The model under review builds one solid part; all positions refer to its coordinate system, in mm. Face numbers are marked on the shaded views. Round coordinates to 2 decimals unless told otherwise and drop trailing zeros. Order: outer loops, then holes, each group sorted by start corner. A loop starts at its lowest first (then second) coordinate and runs counter-clockwise, first axis right, second up. Notation, with made-up numbers: M 18.5,-18.5 L 76.5,-18.5 A31 ccw 76.5,9.5 Z; hole C -31,63.5 d1. An arc over 180 degrees is marked long. Use a Markdown table: item, result. Add a question column.
1. The part is to be moulded in two halves that separate along Y. For the marked faces 1 and 2, say which applies: +Y half, -Y half, draft (parallel to the pull), parting line (faces both ways), or undercut.
2. Consider section A-A on z = 0. State the section outline as (x, y) points.
3. Consider section C-C on y = 12. State the section outline as (x, z) points.
4. Consider section B-B on x = -6. State the section outline as (y, z) points.
5. Insertion check: P1, Ø4, axis at x = 44.5, y = 20, coming from the -Z side; P2, Ø1.2, axis at x = -65.5, y = 2.5, coming from the +Z side; P3, Ø10, axis at x = 21.5, z = 1, coming from the +Y side; P4, Ø10, axis at y = 20, z = 1.5, coming from the -X side. Each pin has a flat end and moves straight along its axis. Give the tip position at first contact, or say it passes through.
6. To check wall thickness, follow probe 1 along X at (y, z) = (3, 0); probe 2 along Y at (x, z) = (41.5, -8.5); probe 3 along Z at (x, y) = (-49, 18). State the ranges of each line that lie inside material, in increasing order.
from build123d import *

# Parameters (mm, degrees)
SKETCH1_W           = 150
SKETCH1_H           = 20
BOSS_EXTRUDE1_DEPTH = 4
BOSS_EXTRUDE3_DEPTH = 150
FILLET1_R           = 4
SKETCH4_W           = 120
SKETCH4_H           = 25.205319461
CUT_EXTRUDE1_DEPTH  = 10
FILLET2_R           = 4
FILLET3_R           = 4
SKETCH6_W           = 124
SKETCH6_H           = 7.02135472
BOSS_EXTRUDE4_DEPTH = 4
BOSS_EXTRUDE5_START = -150
BOSS_EXTRUDE5_DEPTH = 150
SKETCH5_R           = 2.005
CUT_EXTRUDE2_DEPTH  = 10


with BuildPart() as part:
    # Sketch1 → Boss-Extrude1 (new body)
    with BuildSketch(Plane(origin=(0, 0, 0), x_dir=(1, 0, 0), z_dir=(0, 1, 0))):
        Rectangle(SKETCH1_W, SKETCH1_H)
        with BuildLine():
            Line((-67.5, 2.5), (-62.5, 2.5))
            ThreePointArc((-62.5, 2.5), (-60, 0), (-62.5, -2.5))
            Line((-62.5, -2.5), (-67.5, -2.5))
            ThreePointArc((-67.5, -2.5), (-70, 0), (-67.5, 2.5))
        make_face(mode=Mode.SUBTRACT)
        with BuildLine():
            Line((62.5, 2.5), (67.5, 2.5))
            ThreePointArc((67.5, 2.5), (70, 0), (67.5, -2.5))
            Line((67.5, -2.5), (62.5, -2.5))
            ThreePointArc((62.5, -2.5), (60, 0), (62.5, 2.5))
        make_face(mode=Mode.SUBTRACT)
    extrude(amount=BOSS_EXTRUDE1_DEPTH)

    # Sketch3 → Boss-Extrude3 (add)
    with BuildSketch(Plane(origin=(75, 0, 0), x_dir=(0, 0, -1), z_dir=(1, 0, 0))):
        Polygon((-10, 0), (-14, 0), (-10.484132576, 30), (-5.518119877, 29.418005257), (-10, 4), align=None)
    extrude(amount=-BOSS_EXTRUDE3_DEPTH)

    # Fillet1
    fillet1_edges = [part.edges().sort_by_distance(p)[0] for p in [
        (75, 29.709002629, 8.001126226),
        (-75, 29.709002629, 8.001126226),
    ]]
    fillet(fillet1_edges, radius=FILLET1_R)

    # Sketch4 → Cut-Extrude1 (cut)
    with BuildSketch(Plane(origin=(0, 1.618508238, 13.810317987), x_dir=(1, 0, 0), z_dir=(0, 0.11639894850026859, 0.9932025396604823))):
        with Locations((0, 15.973074452)):
            Rectangle(SKETCH4_W, SKETCH4_H)
    extrude(amount=-CUT_EXTRUDE1_DEPTH, mode=Mode.SUBTRACT)

    # Fillet2
    fillet2_edges = [part.edges().sort_by_distance(p)[0] for p in [
        (-60, 29.709002629, 8.001126226),
        (60, 29.709002629, 8.001126226),
    ]]
    fillet(fillet2_edges, radius=FILLET2_R)

    # Fillet3
    fillet3_edges = [part.edges().sort_by_distance(p)[0] for p in [
        (-75, 2, -10),
        (75, 2, -10),
    ]]
    fillet(fillet3_edges, radius=FILLET3_R)

    # Sketch6 → Boss-Extrude4 (add)
    with BuildSketch(Plane(origin=(0, 4, 0), x_dir=(1, 0, 0), z_dir=(0, 1, 0))):
        with Locations((2, -6.973455216)):
            Rectangle(SKETCH6_W, SKETCH6_H)
    extrude(amount=-BOSS_EXTRUDE4_DEPTH)

    # Sketch8 → Boss-Extrude5 (add)
    with BuildSketch(Plane(origin=(75, 0, 0), x_dir=(0, 0, -1), z_dir=(1, 0, 0)).offset(BOSS_EXTRUDE5_START)):
        Polygon((-6.213877267, 25.472169021), (-8.496997767, 4), (-13.531217677, 4), (-10.94972837, 26.027189841), align=None)
    extrude(amount=BOSS_EXTRUDE5_DEPTH)

    # Sketch5 → Cut-Extrude2 (cut)
    with BuildSketch(Plane(origin=(0, 1.618508238, 13.810317987), x_dir=(1, 0, 0), z_dir=(0, 0.11639894850026859, 0.9932025396604823))):
        with Locations(Location((-67.5, 23.575734182, 0), (0, 0, 270))):
            Circle(SKETCH5_R)
        with Locations(Location((67.5, 23.575734182, 0), (0, 0, 270))):
            Circle(SKETCH5_R)
    extrude(amount=-CUT_EXTRUDE2_DEPTH, mode=Mode.SUBTRACT)


solid = part.part
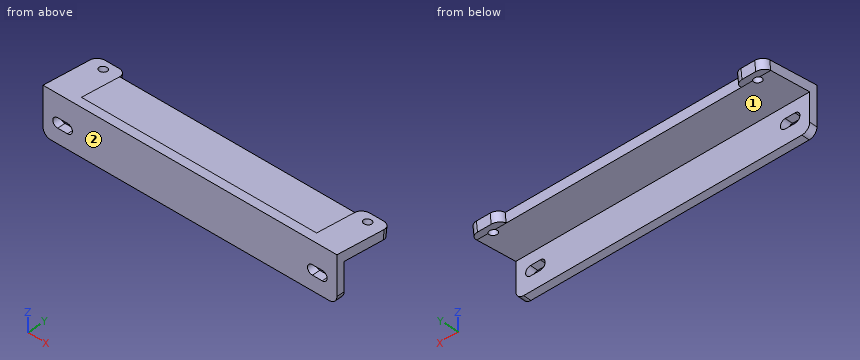
Answer block:
| question | item | result |
|---|---|---|
| 1 | face 1 | undercut |
| 1 | face 2 | -Y half |
| 2 | outline | M -75,0 L -70,0 L -70,4 L -75,4 Z; M -60,0 L 60,0 L 60,4 L -60,4 Z; M 70,0 L 75,0 L 75,4 L 70,4 Z |
| 3 | outline | M -75,7.65 L 75,7.65 L 75,12.59 L -75,12.59 Z |
| 4 | outline | M 0,-10 L 4,-10 L 4,8.5 L 25.47,6.21 L 26.03,10.95 L 0,14 Z |
| 5 | P1 | z = 6.58 |
| 5 | P2 | z = 13.78 |
| 5 | P3 | y = 4 |
| 5 | P4 | through |
| 6 | probe 1 | -75 to -70, -60 to 60, 70 to 75 |
| 6 | probe 2 | 0 to 4 |
| 6 | probe 3 | 7.01 to 11.89 |
